Autodesk Inventor part; units mm, degrees
ref_plane "YZ Plane" through (0, 0, 0) normal (1, 0, 0) x (0, 1, 0)
ref_plane "XZ Plane" through (0, 0, 0) normal (0, 1, 0) x (-1, 0, 0)
ref_plane "XY Plane" through (0, 0, 0) normal (0, 0, 1) x (1, 0, 0)
sketch "Sketch1" plane through (0, 0, 0) normal (0, 0, 1) x (1, 0, 0)
  line L0 (-236.677, 154.5) -> (236.677, 154.5)
  line L1 (236.677, 154.5) -> (236.677, -154.5)
  line L2 (236.677, -154.5) -> (-236.677, -154.5)
  line L3 (-236.677, -154.5) -> (-236.677, 154.5)
  point P0 (0, 0)
  point P1 (0, 154.5)
  point P2 (-236.677, 0)
  dimension "d0" = 473.354
  dimension "d1" = 309
extrude "Extrusion1" add sketch "Sketch1" along normal blind 2
sketch "Sketch2" plane through (0, 0, 2) normal (0, 0, 1) x (1, 0, 0)
  line L0 (-236.677, 154.5) -> (236.677, 154.5)
  line L1 (236.677, 154.5) -> (236.677, -154.5)
  line L2 (236.677, -154.5) -> (-236.677, -154.5)
  line L3 (-236.677, -154.5) -> (-236.677, 154.5)
  line L4 (-234.677, 152.5) -> (234.677, 152.5)
  line L5 (234.677, 152.5) -> (234.677, -152.5)
  line L6 (234.677, -152.5) -> (-234.677, -152.5)
  line L7 (-234.677, -152.5) -> (-234.677, 152.5)
  point P0 (0, 0)
  dimension "d4" = 2
extrude "Extrusion2" add sketch "Sketch2" along normal blind 10
fillet "Fillet1" radius 5 8 edges at (236.677, -154.5, 6) (234.677, -152.5, 7) (-236.677, -154.5, 6) (-234.677, -152.5, 7) (-234.677, 152.5, 7) (236.677, 154.5, 6) (234.677, 152.5, 7) (-236.677, 154.5, 6)
sketch "Sketch4" plane through (0, 0, 0) normal (0, 0, -1) x (-1, 0, 0)
  line L0 (-231.677, -154.5) -> (231.677, -154.5)
  line L1 (236.677, -149.5) -> (236.677, 149.5)
  line L2 (-80.477, 154.5) -> (-130.477, 154.5)
  line L3 (-130.477, 154.5) -> (-130.477, 128.5)
  line L4 (-130.477, 128.5) -> (-80.477, 128.5)
  line L5 (-80.477, 128.5) -> (-80.477, 154.5)
  line L6 (231.677, 154.5) -> (-231.677, 154.5)
  line L7 (-236.677, 149.5) -> (-236.677, -149.5)
  circle A0 centre (-60.807, 122.34) radius 1.5
  circle A1 centre (-160.677, 122.34) radius 1.5
  point P0 (0, 0)
  point P1 (0, 0)
  dimension "d24" = 50
  dimension "d25" = 106.2
  dimension "d26" = 3
  dimension "d27" = 3
  dimension "d28" = 32.16
  dimension "d29" = 99.87
  dimension "d30" = 76
  dimension "d33" = 26
extrude "Extrusion4" cut sketch "Sketch4" against normal blind 5
fillet "Fillet2" radius 3 4 edges at (80.477, 128.5, 1) (130.477, 128.5, 1) (130.477, 153.5, 5) (80.477, 153.5, 5)
properties part number "printer floor plate"
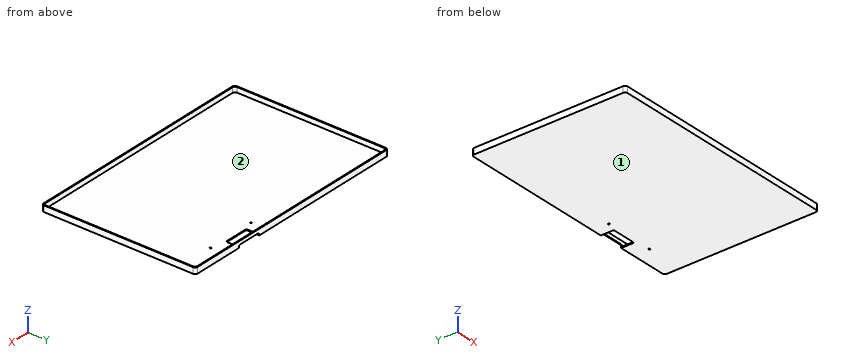
Can you work these out from the model? Positions are in its coordinate system, mm. Face numbers are marked on the shaded views. Coordinates: 2 decimals unless noted, no trailing zeros. Loops run counter-clockwise (first coordinate to the right, second up) from the corner with the lowest first, then second, coordinate; pieces in that order, holes last. Notation, with made-up numbers: (68, 10) - (73, 10) arc R14 ccw to (73, 18) - close; hole circle Ø3 at (33.25, -22). An arc over 180 degrees is marked (long way). Put each result on its own line as item: value. Start each with the question number.
Item 1: Suppose I cut it at B-B (x = -118). Please give me the cut outline in (y, z).
Item 2: Suppose I cut it at A-A (y = -123). Please give me the cut outline in (x, z).
Item 3: If we mould it in two halves opening along X, with no side actions, what happens to the marked faces 1 and 2? For each: +X half, -X half, draft (parallel to the pull), parting line (faces both ways), or undercut.
Item 4: For pin 1 (4 mm diameter, centred on x = 94, y = -109.5, fed in from +Z); pin 2 (1.6 mm diameter, centred on x = 96.5, y = 153.5, fed in from -Z); pin 3 (2.5 mm diameter, centred on x = 160.677, y = 122.34, fed in from -Z); pin 4 (0.6 mm diameter, centred on x = 111.5, z = 1.5, fed in from +Y), each with a flat end and sliding along its axis, tell me the tip position at first contact or that it passes through.
Item 5: If I drill on line 1 along X through (y, z) = (122.34, 1.35); line 2 along X through (y, z) = (-2.5, 2.5); line 3 along Y through (x, z) = (72, 11.25), over which ranges is the centre line in solid material (lowest first)?
Here are the results:
1. outline: (-154.5, 0) - (154.5, 0) - (154.5, 12) - (152.5, 12) - (152.5, 2) - (-152.5, 2) - (-152.5, 12) - (-154.5, 12) - close
2. outline: (-236.68, 0) - (236.68, 0) - (236.68, 12) - (234.68, 12) - (234.68, 2) - (-234.68, 2) - (-234.68, 12) - (-236.68, 12) - close
3. face 1: draft
3. face 2: undercut
4. pin 1: z = 2
4. pin 2: z = 5
4. pin 3: through
4. pin 4: y = 128.5
5. line 1: -236.68 to 59.31, 62.31 to 159.18, 162.18 to 236.68
5. line 2: -236.68 to -234.68, 234.68 to 236.68
5. line 3: -154.5 to -152.5, 152.5 to 154.5
